Geometry: final body of the model. Coordinates: model frame, mm. Give positions to 0.01 mm unless a question says otherwise; leave off trailing zeros. Write each loop counter-clockwise with the first axis right and the second up, starting at its lowest first coordinate (ties: lowest second). Pieces come first, ordered by that corner, then holes. Notation, with made-up numbers: (-20.75, 75.25) -> (4.25, 75.25) arc R24 ccw to (4.25, 85.25) -> close; hole circle Ø8 at (78, 60.5). An arc over 180 degrees is marked (long way). Answer as a JSON object with one key per item and string values.
from build123d import *

# Parameters (mm, degrees)
BOSS_EXTRUDE1_DEPTH = 6
FILLET1_R           = 10


with BuildPart() as part:
    # Sketch1 → Boss-Extrude1 (new body)
    with BuildSketch(Plane(origin=(0, 0, 0), x_dir=(1, 0, 0), z_dir=(0, 1, 0))):
        Polygon((-750, 396), (-690, 396), (-690, 380), (-60, 380), (-60, 396), (0, 396), (0, -16), (-60, -16), (-60, 0), (-690, 0), (-690, -16), (-750, -16), align=None)
    extrude(amount=BOSS_EXTRUDE1_DEPTH)

    # Fillet1
    fillet1_edges = [part.edges().sort_by_distance(p)[0] for p in [
        (-690, 3, -380),
        (-60, 3, -380),
        (-60, 3, 0),
        (-690, 3, 0),
    ]]
    fillet(fillet1_edges, radius=FILLET1_R)


solid = part.part
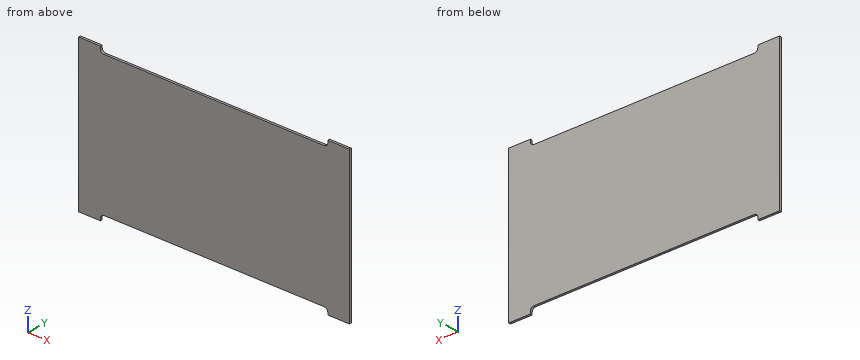
Q1. Cut plane B-B (x = -383). Return the cut outline in (y, z).
Values:
{"outline": "(0, -380) -> (6, -380) -> (6, 0) -> (0, 0) -> close"}
Q2. Material intervals for L1, parallel to Z at x = -521.5, y = 3.1; L2, parallel to Z at x = -685, y = 5.45, sorted ascending. Write a range as from..to.
Values:
{"L1": "-380..0", "L2": "-381.34..1.34"}
Q3. Cut plane A-A (y = 3.35). Return the cut outline in (x, z).
Values:
{"outline": "(-750, -396) -> (-690, -396) -> (-690, -390) arc R10 cw to (-680, -380) -> (-70, -380) arc R10 cw to (-60, -390) -> (-60, -396) -> (0, -396) -> (0, 16) -> (-60, 16) -> (-60, 10) arc R10 cw to (-70, 0) -> (-680, 0) arc R10 cw to (-690, 10) -> (-690, 16) -> (-750, 16) -> close"}
Q4. First-contact query: P1, Ø1, axis at x = -504.5, y = 1, coming from the +Z side. Flat tip, straight axial feed; report the tip coordinate or a pass-through.
Values:
{"P1": "z = 0"}
